Input: part model. Units: mm. Frame: model coordinates. Face numbers are marked on the shaded views. A direction names the side the tool comes from. Coordinates: 2 decimals unless noted, no trailing zeros. Loops run counter-clockwise (first coordinate to the right, second up) from the corner with the lowest first, then second, coordinate; pieces in that order, holes last.
Item 1: Pull-direction query (X, two-part tool) for the marked faces 1 and 2; classes: released by +X, released by -X, zero draft, split by the parting line, or undercut.
Item 2: Section A-A on z = 27.7. Return loops of the section in (x, y).
Item 3: Section C-C on y = 4.5. Return loops of the section in (x, z).
Item 4: Section B-B on x = -19.7. Return loops of the section in (y, z).
Item 5: Section D-D on x = 3.5. Return loops of the section in (y, z).
Item 6: Reachability of the marked faces 3 and 4 from +Z, -Z, +X, -X, +Y, -Y: full face, straight path, thin tool, end or side. Return the list, or none.
Item 7: Contact query for flat-ended pins moving along their axis: P1, Ø2.5, axis at x = 19.7, z = 27.7, coming from the +Y side; P2, Ø2, axis at y = 1.5, z = -6, coming from the -X side; P3, Ø1.1, axis at y = 2, z = 28, coming from the +X side. Output: stop coordinate, or through.
Item 8: Ray query, line 1 along X through (y, z) = (5.75, -25); line 2 along X through (y, z) = (0.6, -27.7); line 3 along X through (y, z) = (4.55, 0). Return the intervals inside material, ascending.
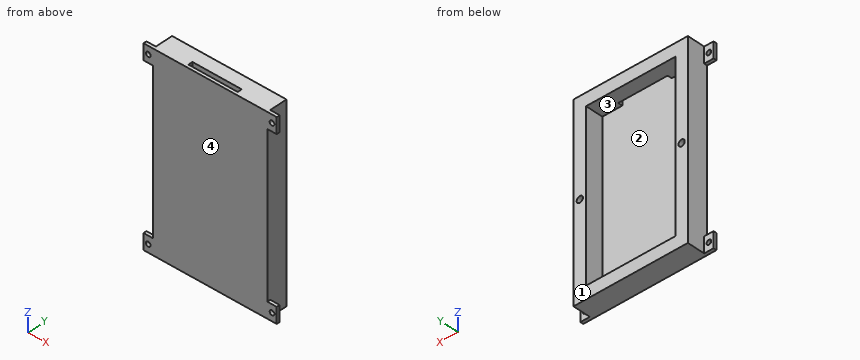
```python
from build123d import *

# Parameters (mm, degrees)
ESBO_O1_W                = 36.4
ESBO_O1_H                = 60.4
ESBO_O1_W_2              = 28.4
ESBO_O1_H_2              = 52.4
RESSALTO_EXTRUS_O1_DEPTH = 6.6
ESBO_O2_W                = 28.4
ESBO_O2_H                = 52.4
RESSALTO_EXTRUS_O2_DEPTH = 1
ESBO_O5_W                = 3
ESBO_O5_H                = 5
ESBO_O5_R                = 0.75
RESSALTO_EXTRUS_O3_DEPTH = 1
ESBO_O6_R                = 1
CORTE_EXTRUS_O3_DEPTH    = 4
ESBO_O3_W                = 15.7
ESBO_O3_H                = 1.4
CORTE_EXTRUS_O4_DEPTH    = 5


with BuildPart() as part:
    # Esboço1 → Ressalto-extrusão1 (new body)
    with BuildSketch(Plane(origin=(0, 0, 0), x_dir=(1, 0, 0), z_dir=(0, 1, 0))):
        Rectangle(ESBO_O1_W, ESBO_O1_H)
        Rectangle(ESBO_O1_W_2, ESBO_O1_H_2, mode=Mode.SUBTRACT)
    extrude(amount=RESSALTO_EXTRUS_O1_DEPTH)

    # Esboço2 → Ressalto-extrusão2 (add)
    with BuildSketch(Plane(origin=(0, 0, 0), x_dir=(1, 0, 0), z_dir=(0, 1, 0))):
        Rectangle(ESBO_O2_W, ESBO_O2_H)
    extrude(amount=RESSALTO_EXTRUS_O2_DEPTH)

    # Esboço5 → Ressalto-extrusão3 (add)
    # profile 1 of 4: a face of its own
    with BuildSketch(Plane(origin=(0, 0, 0), x_dir=(1, 0, 0), z_dir=(0, 1, 0))):
        with Locations((-19.7, 27.7)):
            Rectangle(ESBO_O5_W, ESBO_O5_H)
        with Locations(Location((-19.7, 27.7, 0), (0, 0, 270))):
            Circle(ESBO_O5_R, mode=Mode.SUBTRACT)
    # profile 2 of 4: a face of its own
    with BuildSketch(Plane(origin=(0, 0, 0), x_dir=(1, 0, 0), z_dir=(0, 1, 0))):
        with Locations((-19.7, -27.7)):
            Rectangle(ESBO_O5_W, ESBO_O5_H)
        with Locations(Location((-19.7, -27.7, 0), (0, 0, 270))):
            Circle(ESBO_O5_R, mode=Mode.SUBTRACT)
    # profile 3 of 4: a face of its own
    with BuildSketch(Plane(origin=(0, 0, 0), x_dir=(1, 0, 0), z_dir=(0, 1, 0))):
        with Locations((19.7, -27.7)):
            Rectangle(ESBO_O5_W, ESBO_O5_H)
        with Locations(Location((19.7, -27.7, 0), (0, 0, 270))):
            Circle(ESBO_O5_R, mode=Mode.SUBTRACT)
    # profile 4 of 4: a face of its own
    with BuildSketch(Plane(origin=(0, 0, 0), x_dir=(1, 0, 0), z_dir=(0, 1, 0))):
        with Locations((19.7, 27.7)):
            Rectangle(ESBO_O5_W, ESBO_O5_H)
        with Locations(Location((19.7, 27.7, 0), (0, 0, 270))):
            Circle(ESBO_O5_R, mode=Mode.SUBTRACT)
    extrude(amount=RESSALTO_EXTRUS_O3_DEPTH)

    # Esboço6 → Corte-extrusão3 (cut)
    with BuildSketch(Plane(origin=(0, 6.6, 0), x_dir=(1, 0, 0), z_dir=(0, 1, 0))):
        with Locations(Location((-16.2, 0, 0), (0, 0, 270))):
            Circle(ESBO_O6_R)
        with Locations(Location((16.2, 0, 0), (0, 0, 270))):
            Circle(ESBO_O6_R)
    extrude(amount=-CORTE_EXTRUS_O3_DEPTH, mode=Mode.SUBTRACT)

    # Esboço3 → Corte-extrusão4 (cut)
    with BuildSketch(Plane.XY.offset(30.2)):
        with Locations((0, 1.7)):
            Rectangle(ESBO_O3_W, ESBO_O3_H)
    extrude(amount=-CORTE_EXTRUS_O4_DEPTH, mode=Mode.SUBTRACT)


solid = part.part
```
Results found:
1. face 1: zero draft
1. face 2: undercut
2. outline: (-21.2, 0) - (-20.45, 0) - (-20.45, 1) - (-21.2, 1) - close; (-18.95, 0) - (18.95, 0) - (18.95, 1) - (18.2, 1) - (18.2, 6.6) - (-18.2, 6.6) - (-18.2, 1) - (-18.95, 1) - close; (20.45, 0) - (21.2, 0) - (21.2, 1) - (20.45, 1) - close; hole (-7.85, 1) - (7.85, 1) - (7.85, 2.4) - (-7.85, 2.4) - close
3. outline: (-18.2, -30.2) - (18.2, -30.2) - (18.2, 30.2) - (-18.2, 30.2) - close; hole circle Ø2 at (-16.2, 0); hole (-14.2, -26.2) - (14.2, -26.2) - (14.2, 26.2) - (-14.2, 26.2) - close; hole circle Ø2 at (16.2, 0)
4. outline: (0, -30.2) - (1, -30.2) - (1, -28.45) - (0, -28.45) - close; (0, -26.95) - (1, -26.95) - (1, -25.2) - (0, -25.2) - close; (0, 25.2) - (1, 25.2) - (1, 26.95) - (0, 26.95) - close; (0, 28.45) - (1, 28.45) - (1, 30.2) - (0, 30.2) - close
5. outline: (0, -30.2) - (6.6, -30.2) - (6.6, -26.2) - (1, -26.2) - (1, 30.2) - (0, 30.2) - close; (2.4, 26.2) - (6.6, 26.2) - (6.6, 30.2) - (2.4, 30.2) - close
6. face 3: +Y
6. face 4: +Z, -Z, +X, -X, -Y
7. P1: stops at y = 1
7. P2: stops at x = -18.2
7. P3: stops at x = 18.2
8. line 1: x = -18.2 to -14.2, 14.2 to 18.2
8. line 2: x = -21.2 to -20.45, -18.95 to 18.95, 20.45 to 21.2
8. line 3: x = -18.2 to -17.2, -15.2 to -14.2, 14.2 to 15.2, 17.2 to 18.2
